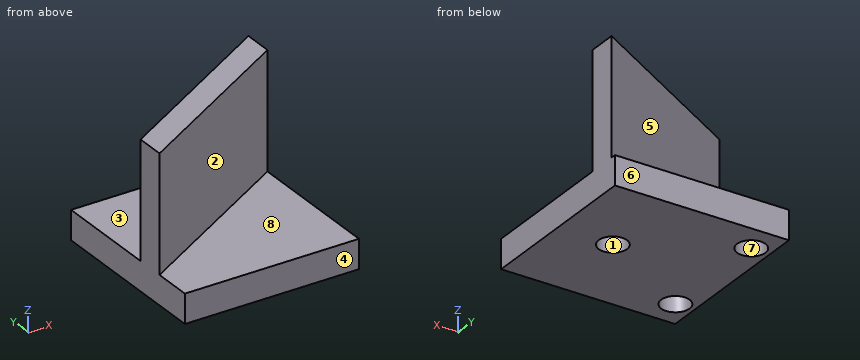
Autodesk Inventor part; units mm, degrees
ref_plane "YZ Plane" through (0, 0, 0) normal (1, 0, 0) x (0, 1, 0)
ref_plane "XZ Plane" through (0, 0, 0) normal (0, 1, 0) x (-1, 0, 0)
ref_plane "XY Plane" through (0, 0, 0) normal (0, 0, 1) x (1, 0, 0)
ref_plane "Arbeitsebene1" through (0, 0, 4) normal (0, 0, 1) x (1, 0, 0)
sketch "Skizze1" plane through (0, 0, 4) normal (0, 0, 1) x (1, 0, 0)
  circle A0 centre (33.0405, -20.0687) radius 1.4
  circle A1 centre (15.72, -10.0687) radius 1.4
  circle A2 centre (15.72, -30.0687) radius 1.4
  line L0 (0, -18.4687) -> (28.3951, -18.4687)
  arc A3 (28.3951, -21.6687) -> (28.3951, -18.4687) centre (28.3951, -20.0687) ccw
  line L1 (28.3951, -21.6687) -> (0, -21.6687)
  line L2 (0, -36.0687) -> (0, -21.6687)
  line L3 (0, -36.0687) -> (55, -36.0687)
  line L4 (55, -36.0687) -> (55, -6.0687)
  line L5 (55, -6.0687) -> (60, -6.0687)
  line L6 (60, 0) -> (60, -6.0687)
  line L7 (0, 0) -> (60, 0)
  line L8 (0, -18.4687) -> (0, 0)
  line L9 (12.5, -35.0687) -> (42.5, -35.0687)
  line L10 (42.5, -35.0687) -> (42.5, -5.0687)
  line L11 (42.5, -5.0687) -> (12.5, -5.0687)
  line L12 (12.5, -5.0687) -> (12.5, -35.0687)
  line L13 (12.5, -35.0687) -> (42.5, -5.0687) construction
  line L14 (42.5, -35.0687) -> (12.5, -5.0687) construction
  circle A4 centre (33.0405, -20.0687) radius 2.45
  circle A5 centre (15.72, -10.0687) radius 2.45
  circle A6 centre (15.72, -30.0687) radius 2.45
  line L15 (12.5, -18.4687) -> (12.5, -21.6687)
  point P0 (27.5, -20.0687)
  point P1 (18.7387, -21.6687)
  point P2 (11.6841, -36.0687)
  point P3 (46.6841, -36.0687)
  point P4 (18.7387, -18.4687)
  dimension "d0" = 30
  dimension "d1" = 30
  dimension "d2" = 4.9
  dimension "d3" = 4.9
  dimension "d4" = 4.9
extrude "Extrusion1" add sketch "Skizze1" along normal blind 4 contours L12 L11 L10 L9 L1 A3 L0 | L0 A3 L1 L12
sketch "Skizze2" plane through (0, 0, 8) normal (0, 0, 1) x (1, 0, 0)
  line L0 (12.5, -5.0687) -> (12.5, -35.0687)
  line L1 (42.5, -35.0687) -> (42.5, -5.0687)
  line L2 (42.5, -5.0687) -> (12.5, -5.0687)
  circle A0 centre (33.0405, -20.0687) radius 2.45
  line L3 (12.5, -35.0687) -> (42.5, -35.0687)
  point P0 (0, 0)
extrude "Extrusion2" add sketch "Skizze2" along normal blind 1 contours L2 L1 L3 L0 | A0
sketch "Skizze3" plane through (0, 0, 9) normal (0, 0, 1) x (1, 0, 0)
  line L0 (12.5, -35.0687) -> (42.5, -35.0687)
  line L1 (42.5, -35.0687) -> (42.5, -5.0687)
  line L2 (42.5, -5.0687) -> (12.5, -5.0687)
  line L3 (12.5, -5.0687) -> (12.5, -35.0687)
  line L4 (37.9557, 14.9579) -> (17.8567, -20.2718)
  line L5 (17.8567, -20.2718) -> (-3.0822, -20.2721)
  line L6 (15.4322, -16.0975) -> (22.0334, -27.4633)
  line L7 (12.5, -5.0687) -> (12.5, -35.0687)
  line L8 (12.5, -23.3829) -> (44.0331, -5.0687)
  line L9 (42.5, -35.0687) -> (42.5, -5.0687)
  line L10 (42.5, -5.9591) -> (42.5, -10.9591)
  line L11 (42.5, -10.9591) -> (12.5, -28.3829)
  point P0 (0, 0)
  point P1 (42.5, -5.9591)
  point P2 (12.5, -28.3829)
  dimension "d9" = 119.706
  dimension "d10" = 59.853
  dimension "d11" = 5
extrude "Extrusion3" add sketch "Skizze3" along normal blind 20 contours L3 L8 L6 L11 | L11 L6 L8 L1
equation "\"d10\" = 0.5 * d9"
properties part number "cellSTORM_Flipmirror"
Source: CAD feature listing. Evaluate the final solid. Frame: model axes, mm. Face numbers are marked on the shaded views. A direction names the side the tool comes from. Coordinates: 2 decimals unless noted, no trailing zeros. Order: outer loops, then holes, each group sorted by start corner. A loop starts at its lowest first (then second) coordinate and runs counter-clockwise, first axis right, second up. Notation, with made-up numbers: (54, 73.25) - (104, 73.25) arc R17 ccw to (104, 102.25) - close; hole circle Ø2 at (12, -36). An arc over 180 degrees is marked (long way). One line per item, written item: value.
1) Cut plane D-D on x = 22.25. Output: boundary loops of the cut face in (y, z), plus the area to 3 significant figures.
Computed values:
outline: (-35.07, 4) - (-5.07, 4) - (-5.07, 9) - (-17.72, 9) - (-17.72, 29) - (-22.72, 29) - (-22.72, 9) - (-35.07, 9) - close
area: 250 mm^2
2) Cut plane A-A on z = 7.25. Output: boundary loops of the cut face in (x, y), plus the area to 3 significant figures.
Computed values:
outline: (12.5, -35.07) - (42.5, -35.07) - (42.5, -5.07) - (12.5, -5.07) - close; hole circle Ø4.9 at (15.72, -30.07); hole circle Ø4.9 at (15.72, -10.07); hole circle Ø4.9 at (33.04, -20.07)
area: 843 mm^2
3) Cut plane C-C on x = 15.72. Output: boundary loops of the cut face in (y, z).
Computed values:
outline: (-35.07, 4) - (-32.52, 4) - (-32.52, 8) - (-27.62, 8) - (-27.62, 4) - (-12.52, 4) - (-12.52, 8) - (-7.62, 8) - (-7.62, 4) - (-5.07, 4) - (-5.07, 9) - (-21.51, 9) - (-21.51, 29) - (-26.51, 29) - (-26.51, 9) - (-35.07, 9) - close
4) Reachability of the marked faces 4, 5, 6, 7 and 8 from +Z, -Z, +X, -X, +Y, -Y: full face, straight path, thin tool, end or side. Return the list, or none.
Computed values:
face 4: +Z, -Z, +X, -X, -Y
face 5: +Z, -X, +Y
face 6: +Z, -Z, +X, -X, +Y
face 7: -Z
face 8: +Z, +X, -Y
5) Mould query, pull axis Y, two halves, no side actions, for the marked faces 1, 2 and 3. Classes: released by +Y, released by -Y, zero draft, split by the parting line, or undercut.
Computed values:
face 1: undercut
face 2: released by -Y
face 3: zero draft
6) Ray query, line 1 (Y direction, x = 15.72, z = 5.1); line 2 (Z direction, x = 40, y = -15); line 3 (Z direction, x = 14.25, y = -10). Return the intervals inside material, ascending. Write a range as [from, to].
Computed values:
line 1: y = [-35.07, -32.52], [-27.62, -12.52], [-7.62, -5.07]
line 2: z = [4, 9]
line 3: z = [8, 9]
7) Cut plane B-B on y = -16.25. Output: boundary loops of the cut face in (x, z).
Computed values:
outline: (12.5, 4) - (42.5, 4) - (42.5, 9) - (33.39, 9) - (33.39, 29) - (24.78, 29) - (24.78, 9) - (12.5, 9) - close
8) Contact query for flat-ended pins moving along their axis: pin 1 (4.5 mm diameter, centred on x = 33.04, y = -20.07, fed in from +Z); pin 2 (4 mm diameter, centred on x = 34.5, z = 12, fed in from +Y); pin 3 (1 mm diameter, centred on x = 32.5, z = 21, fed in from +Y). Output: stop coordinate, or through.
Computed values:
pin 1: stops at z = 9
pin 2: stops at y = -9.44
pin 3: stops at y = -11.48
